Source: CAD feature listing. Evaluate the final solid. Frame: model axes, mm. A direction names the side the tool comes from. Round coordinates to 2 decimals unless told otherwise and drop trailing zeros. Loops run counter-clockwise (first coordinate to the right, second up) from the corner with the lowest first, then second, coordinate; pieces in that order, holes last.
(1) First-contact query: pin 1 Ø2 at (y, z) = (-2.5, 17) entering from -X; pin 2 Ø3 at (x, z) = (-0.5, 56.5) entering from +Y. Flat tips, straight axial feed; report the tip coordinate or a pass-through.
(2) Mould query, pull axis Z, two halves, no side actions, for faces 1 (the conical face through (-2.09, -0.46, 147.86)), 2 (the cylindrical face through (1.62, 0.51, 71.48)), 3 (the flat face through (-1, 0, 0)). Classes: pulls with the +Z half, pulls with the -Z half, needs draft (parallel to the pull), parting line crosses it, or undercut.
(3) Set-up query: faces 4 (the flat face through (-1, 0, 150)), 5 (the flat face through (-1.4, 1.4, 145)), 6 (the cylindrical face through (1.62, 0.51, 149.49)). Return all of +Z, -Z, +X, -X, +Y, -Y with unobstructed straight access to the full face (end or side cutting, diameter ignored); none if empty.
(4) Material intervals for probe 1 along Y at (x, z) = (0, 117); probe 2 along Y at (x, z) = (-0.5, 68), sorted ascending.
(5) Section A-A, the plane z = 104. Return the cut outline in (x, y), plus the area to 3 significant figures.
```python
from build123d import *

# Parameters (mm, degrees)
SKETCH1_R           = 1.7
SKETCH1_R_2         = 0.85
BOSS_EXTRUDE1_DEPTH = 150


with BuildPart() as part:
    # Sketch1 → Boss-Extrude1 (new body)
    with BuildSketch(Plane.XY):
        Circle(SKETCH1_R)
        Circle(SKETCH1_R_2, mode=Mode.SUBTRACT)
    extrude(amount=BOSS_EXTRUDE1_DEPTH)

    # Sketch3 → Revolve1 (revolve)
    with BuildSketch(Plane(origin=(0, 0, 0), x_dir=(0, 0, -1), z_dir=(1, 0, 0))):
        Polygon((-149, 1.7), (-145, 3.25), (-145, 1.7), align=None)
    revolve(axis=Axis((0, 0, 150), (0, 0, -1)))


solid = part.part
```
Output values:
1. pin 1: stops at x = -0.8
1. pin 2: stops at y = 1.7
2. face 1: pulls with the +Z half
2. face 2: needs draft
2. face 3: pulls with the -Z half
3. face 4: +Z, +X, -X, +Y, -Y
3. face 5: -Z
3. face 6: +Z
4. probe 1: y = -1.7 to -0.85, 0.85 to 1.7
4. probe 2: y = -1.62 to -0.69, 0.69 to 1.62
5. outline: circle Ø3.4 at (0, 0); hole circle Ø1.7 at (0, 0)
5. area: 6.81 mm2
